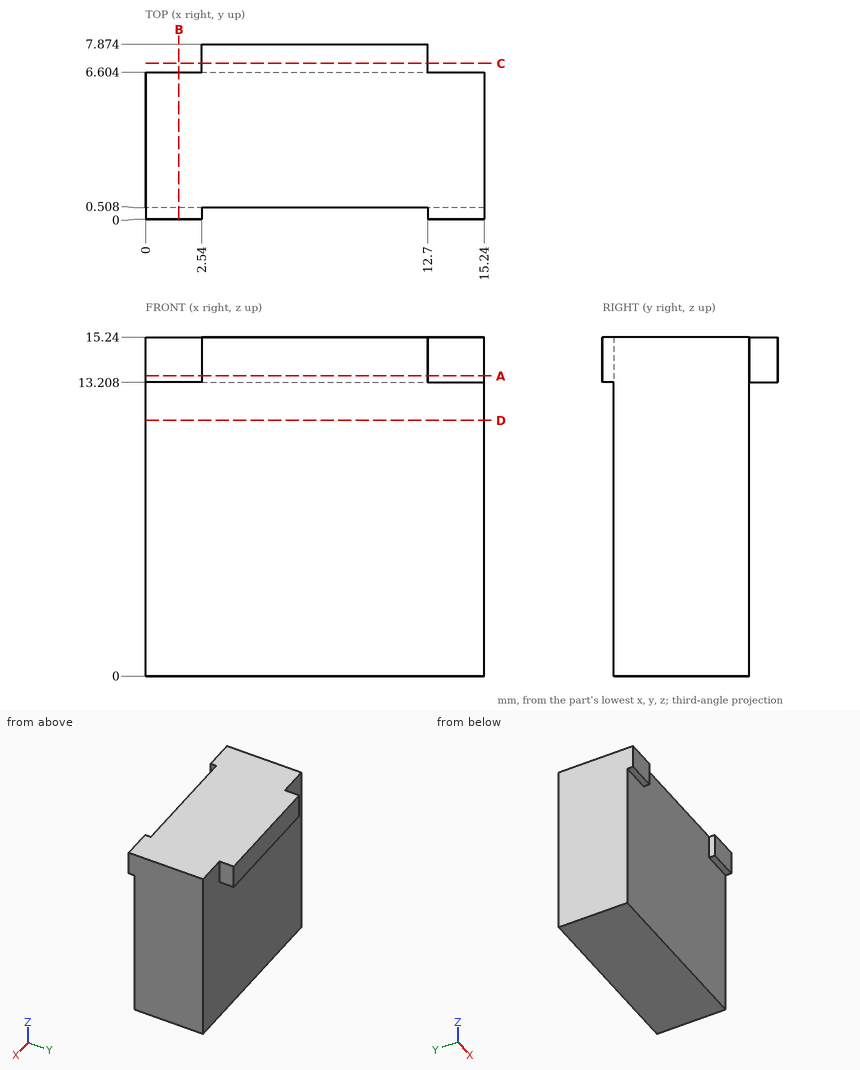
Drawing for the job (mm, zero at the part's lowest x, y, z). Round coordinates to 2 decimals unless told otherwise and drop trailing zeros. Order: outer loops, then holes, each group sorted by start corner. A loop starts at its lowest first (then second) coordinate and runs counter-clockwise, first axis right, second up.
Item 1: Saw through at D-D on z = 11.5. Write the cut outline in (x, y), then the cut area to 3 significant figures.
Item 2: Probe line 1 along Y through (x, z) = (11.5, 3.5). List the from-to ranges inside material, lowest first.
Item 3: Pin check, flat tip, straight feed: pin 1 (4.5 mm diameter, centred on x = 10, z = 5, fed in from +Y). Stop position of the tip, or through.
Item 4: Saw through at A-A on z = 13.5. Write the cut outline in (x, y), then the cut area to 3 significant figures.
Item 5: Saw through at B-B on x = 1.5. Write the cut outline in (y, z).
Item 6: Saw through at C-C on y = 7. Write the cut outline in (x, z), then the cut area to 3 significant figures.
Reported:
1. outline: (0, 0.51) - (15.24, 0.51) - (15.24, 6.6) - (0, 6.6) - close
1. area: 92.9 mm2
2. line 1: y = 0.51 to 6.6
3. pin 1: stops at y = 6.6
4. outline: (0, 0) - (2.54, 0) - (2.54, 0.51) - (12.7, 0.51) - (12.7, 0) - (15.24, 0) - (15.24, 6.6) - (12.7, 6.6) - (12.7, 7.87) - (2.54, 7.87) - (2.54, 6.6) - (0, 6.6) - close
4. area: 108 mm2
5. outline: (0, 13.21) - (0.51, 13.21) - (0.51, 0) - (6.6, 0) - (6.6, 15.24) - (0, 15.24) - close
6. outline: (2.54, 13.21) - (12.7, 13.21) - (12.7, 15.24) - (2.54, 15.24) - close
6. area: 20.6 mm2
